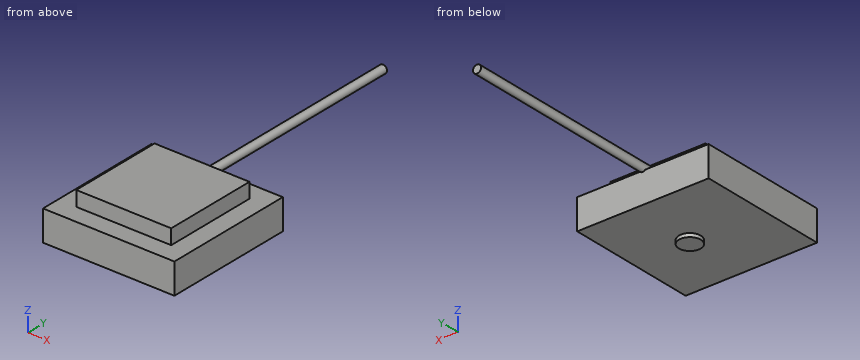
from build123d import *

# Parameters (mm, degrees)
SKETCH1_W           = 18
SKETCH1_H           = 18
BOSS_EXTRUDE1_DEPTH = 4.15
SKETCH2_W           = 13
SKETCH2_H           = 13
BOSS_EXTRUDE2_DEPTH = 2.05
SKETCH3_R           = 1.5
BOSS_EXTRUDE3_DEPTH = 0.5
SKETCH4_R           = 0.551632399
BOSS_EXTRUDE4_DEPTH = 30


with BuildPart() as part:
    # Sketch1 → Boss-Extrude1 (new body)
    with BuildSketch(Plane.XY):
        with Locations((9, 9)):
            Rectangle(SKETCH1_W, SKETCH1_H)
    extrude(amount=BOSS_EXTRUDE1_DEPTH)

    # Sketch2 → Boss-Extrude2 (add)
    with BuildSketch(Plane.XY.offset(4.15)):
        with Locations((9, 9)):
            Rectangle(SKETCH2_W, SKETCH2_H)
    extrude(amount=BOSS_EXTRUDE2_DEPTH)

    # Sketch3 → Boss-Extrude3 (add)
    with BuildSketch(Plane(origin=(0, 0, 0), x_dir=(-1, 0, 0), z_dir=(0, 0, -1))):
        with Locations((-10, 9)):
            Circle(SKETCH3_R)
    extrude(amount=BOSS_EXTRUDE3_DEPTH)

    # Sketch4 → Boss-Extrude4 (add)
    with BuildSketch(Plane(origin=(0, 15.5, 0), x_dir=(1, 0, 0), z_dir=(0, 1, 0))):
        with Locations(Location((9.049626603, -4.551632399, 0), (0, 0, 133.274343649))):
            Circle(SKETCH4_R)
    extrude(amount=BOSS_EXTRUDE4_DEPTH)


solid = part.part
Can you work these out from the model? Positions are in its coordinate system, mm. Round coordinates to 2 decimals unless told otherwise and drop trailing zeros. Loops run counter-clockwise (first coordinate to the right, second up) from the corner with the lowest first, then second, coordinate; pieces in that order, holes last. Notation, with made-up numbers: (79.25, 57) - (110.25, 57) arc R26 cw to (110.25, 76) - close; hole circle Ø11 at (29.5, 43.5). An arc over 180 degrees is marked (long way). Use CSV: the item, a comma, the result in double quotes. Start each with the question number.
1) If we section it at C-C on z = 3.5: Write out the boundary of the cut face in (x, y).
2) If we section it at A-A on y = 13: Write out the boundary of the cut face in (x, z).
3) If we section it at D-D on x = 10: Write out the boundary of the cut face in (y, z), plus the area to 3 significant figures.
4) Please list where these lines run through material, in increasing order: probe 1 along Z at (x, y) = (8.5, 8); probe 2 along Y at (x, z) = (15.5, 1.5); probe 3 along Y at (x, z) = (7.5, 6). Write a range as [from, to].
5) For pin 1 Ø0.6 at (x, z) = (7.5, 5) entering from +Y; pin 2 Ø3 at (x, z) = (4.5, 4.5) entering from +Y; pin 3 Ø1 at (x, z) = (6, 5) entering from -Y; pin 4 Ø1 at (x, y) = (11, 33) entering from -Z, each with a flat end and sliding along its axis, tell me the tip position at first contact or that it passes through.
Geometry results:
1,outline,"(0, 0) - (18, 0) - (18, 18) - (0, 18) - close"
2,outline,"(0, 0) - (18, 0) - (18, 4.15) - (15.5, 4.15) - (15.5, 6.2) - (2.5, 6.2) - (2.5, 4.15) - (0, 4.15) - close"
3,outline,"(0, 0) - (7.5, 0) - (7.5, -0.5) - (10.5, -0.5) - (10.5, 0) - (18, 0) - (18, 4.15) - (15.5, 4.15) - (15.5, 6.2) - (2.5, 6.2) - (2.5, 4.15) - (0, 4.15) - close"
3,area,"103 mm2"
4,probe 1,"z = [0, 6.2]"
4,probe 2,"y = [0, 18]"
4,probe 3,"y = [2.5, 15.5]"
5,pin 1,"stops at y = 15.5"
5,pin 2,"stops at y = 18"
5,pin 3,"stops at y = 2.5"
5,pin 4,"passes through"
